Here's how the part is built. I have some questions about the finished solid (model axes, mm). Face numbers are marked on the shaded views. A direction names the side the tool comes from. Round coordinates to 2 decimals unless told otherwise and drop trailing zeros. Order: outer loops, then holes, each group sorted by start corner. A loop starts at its lowest first (then second) coordinate and runs counter-clockwise, first axis right, second up.
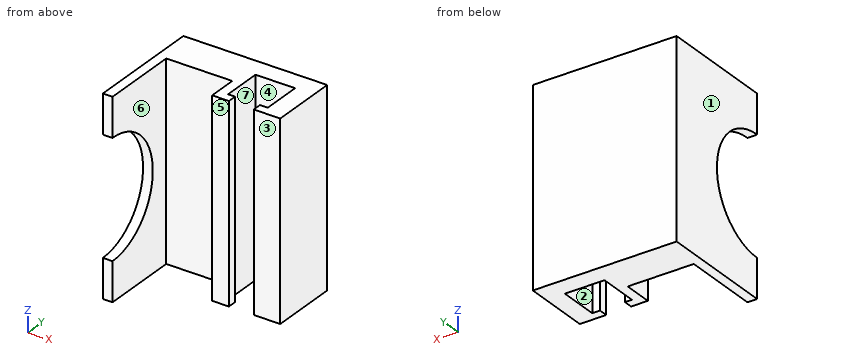
Autodesk Inventor part; units mm, degrees
ref_plane "YZ Plane" through (0, 0, 0) normal (1, 0, 0) x (0, 1, 0)
ref_plane "XZ Plane" through (0, 0, 0) normal (0, 1, 0) x (-1, 0, 0)
ref_plane "XY Plane" through (0, 0, 0) normal (0, 0, 1) x (1, 0, 0)
sketch "Skizze1" plane through (0, 0, 0) normal (0, 0, 1) x (1, 0, 0)
  line L0 (0, 0) -> (22, 0)
  line L1 (22, 0) -> (22, 10)
  line L2 (22, 10) -> (0, 10)
  line L3 (0, 10) -> (0, 0)
  dimension "d0" = 22
  dimension "d1" = 10
extrude "Extrusion1" add sketch "Skizze1" along normal blind 50
sketch "Skizze3" plane through (22, 0, 0) normal (1, 0, 0) x (0, 0, -1)
  line L0 (-50, 0) -> (-50, 10)
  line L1 (0, 0) -> (0, 10)
  line L2 (-50, 10) -> (0, 10)
  line L3 (0, 10) -> (0, 5)
  line L4 (0, 5) -> (-50, 5)
  line L5 (-50, 5) -> (-50, 10)
extrude "Extrusion2" add sketch "Skizze3" along normal blind 15
sketch "Skizze4" plane through (22, 5, 0) normal (0, -1, 0) x (1, 0, 0)
  line L0 (-22, 50) -> (15, 50)
  line L1 (15, 50) -> (10.2, 50)
  line L2 (10.2, 50) -> (10.2, 0)
  line L3 (10.2, 0) -> (15, 0)
  line L4 (15, 0) -> (15, 50)
  line L5 (0, 0) -> (0, 50)
  point P0 (-22, 0)
  dimension "d6" = 10.2
extrude "Extrusion3" add sketch "Skizze4" along normal blind 5
sketch "Skizze5" plane through (0, 0, 0) normal (0, -1, 0) x (1, 0, 0)
  line L0 (22, 0) -> (22, 50)
  line L1 (22, 50) -> (17, 50)
  line L2 (17, 50) -> (17, 0)
  line L3 (17, 0) -> (22, 0)
  line L4 (22, 0) -> (22, 50)
  line L5 (32.2, 50) -> (32.2, 0)
  line L6 (37, 0) -> (37, 50)
  line L7 (32.2, 50) -> (37, 50)
  line L8 (37, 50) -> (37, 0)
  line L9 (37, 0) -> (32.2, 0)
  line L10 (32.2, 0) -> (32.2, 50)
  point P0 (0, 0)
  dimension "d9" = 5
extrude "Extrusion4" add sketch "Skizze5" along normal blind 10
sketch "Skizze6" plane through (32.2, 5, 0) normal (-1, 0, 0) x (0, 0, 1)
  line L0 (50, 5) -> (50, -15)
  line L1 (0, 5) -> (0, -15)
  line L2 (50, -15) -> (0, -15)
  line L3 (0, -15) -> (0, -10.2)
  line L4 (0, -10.2) -> (50, -10.2)
  line L5 (50, -10.2) -> (50, -15)
  point P0 (0, -5)
  point P1 (0, -15)
  point P2 (50, -10.2)
  dimension "d12" = 4.8
extrude "Extrusion5" add sketch "Skizze6" along normal blind 2
ref_plane "Arbeitsebene1" through (27, 0, 0) normal (-1, 0, 0) x (0, 0, 1)
mirror "Spiegeln1" about plane through (27, 0, 0) normal (-1, 0, 0) of "Extrusion5"
sketch "Skizze7" plane through (0, -10, 0) normal (0, -1, 0) x (1, 0, 0)
  line L0 (0, 50) -> (37, 50)
  line L1 (17, 0) -> (17, 50)
  line L2 (37, 50) -> (17, 50)
  line L3 (17, 50) -> (17, 0)
  line L4 (17, 0) -> (37, 0)
  line L5 (37, 0) -> (37, 50)
  point P0 (0, 0)
extrude "Extrusion6" cut sketch "Skizze7" against normal blind 2.5
sketch "Skizze8" plane through (0, 0, 0) normal (-1, 0, 0) x (0, 0, 1)
  point P0 (0, 0)
sketch "Skizze9" plane through (0, 0, 0) normal (-1, 0, 0) x (0, 0, 1)
  line L0 (50, -20) -> (0, -20)
  line L1 (0, -20) -> (0, 30)
  line L2 (0, 30) -> (50, 30)
  line L3 (50, 30) -> (50, -20)
  line L4 (0, 0) -> (50, 0)
  line L5 (50, 10) -> (50, 0)
  point P0 (50, 5)
  dimension "d17" = 50
  dimension "d18" = 50
  dimension "d19" = 20
  dimension "d20" = 0
extrude "Extrusion7" add sketch "Skizze9" against normal blind 2.5
sketch "Skizze10" plane through (0, -20, 0) normal (-1, 0, 0) x (0, 0, 1)
  circle A0 centre (25, 0) radius 15
  line L0 (0, 0) -> (50, 0)
  point P0 (0, 20)
  point P1 (25, 0)
  point P2 (10, 0)
  point P3 (40, 0)
  dimension "d23" = 30
extrude "Extrusion8" cut sketch "Skizze10" against normal blind 2.5 contours L0 A0 picked at (21.7322, 7.6351)
sketch "Skizze11" plane through (17, 0, 0) normal (-1, 0, 0) x (0, 0, 1)
  line L0 (0, -7.5) -> (50, -7.5)
  line L1 (0, 0) -> (0, -7.5)
  line L2 (50, -7.5) -> (0, -7.5)
  line L3 (0, -7.5) -> (0, 0)
  line L4 (0, 0) -> (50, 0)
  line L5 (50, 0) -> (50, -7.5)
extrude "Extrusion9" cut sketch "Skizze11" against normal blind 2.5
sketch "Skizze12" plane through (2.5, 0, 0) normal (1, 0, 0) x (0, 0, -1)
  line L0 (-50, 10) -> (-50, -7.5)
  line L1 (0, 30) -> (0, -20)
  line L2 (-50, 10) -> (0, 10)
  line L3 (0, 10) -> (0, 30)
  line L4 (0, 30) -> (-50, 30)
  line L5 (-50, 30) -> (-50, 10)
  point P0 (0, 0)
  point P1 (0, 10)
extrude "Extrusion10" cut sketch "Skizze12" against normal blind 10
properties part number "Schiene"
1. If we section it at C-C, the plane z = 34: Write out the boundary of the cut face in (x, y), and give its area (3 significant figures).
Evaluation:
outline: (0, -8) - (2.5, -8) - (2.5, 0) - (19.5, 0) - (19.5, -7.5) - (23.8, -7.5) - (23.8, -5.2) - (22, -5.2) - (22, 5) - (32.2, 5) - (32.2, -5.2) - (30.2, -5.2) - (30.2, -7.5) - (37, -7.5) - (37, 10) - (0, 10) - close
area: 402 mm2
2. I'm going to push flat-ended pins straight in: P1, Ø5, axis at x = 29, z = 23, coming from the -Y side; P2, Ø5, axis at x = 9.5, z = 20, coming from the -Y side. Where does each tip first touch, or does it pass through?
Evaluation:
P1: stops at y = -7.5
P2: stops at y = 0
3. I need wall thicknesses on probe 1 along X at (y, z) = (-7, 4); probe 2 along X at (y, z) = (3, 14); probe 3 along Y at (x, z) = (22.5, 14). Which ranges of each line are inside material? Lowest first, please.
Evaluation:
probe 1: x = 0 to 2.5, 19.5 to 23.8, 30.2 to 37
probe 2: x = 0 to 22, 32.2 to 37
probe 3: y = -7.5 to -5.2, 5 to 10
4. If we mould it in two halves opening along Y, with no side actions, what happens to the marked faces 1, 2, 3 and 4? For each: released by +Y, released by -Y, zero draft, split by the parting line, or undercut.
Evaluation:
face 1: zero draft
face 2: undercut
face 3: released by -Y
face 4: undercut
5. On a 3-axis mill with a long thin cutter (end or side, diameter ignored), from which of +Z, -Z, +X, -X, +Y, -Y can I reach the whole of each face in a straight line? I mean the marked faces 5, 6 and 7. Say none if no direction works.
Evaluation:
face 5: +Z, -Z, +X, -Y
face 6: +Z, -Z, -Y
face 7: +Z, -Z
6. If we section it at B-B, the plane y = 4: Write out the boundary of the cut face in (x, z), and give its area (3 significant figures).
Evaluation:
outline: (0, 0) - (22, 0) - (22, 50) - (0, 50) - close; (32.2, 0) - (37, 0) - (37, 50) - (32.2, 50) - close
area: 1,340 mm2
7. If we section it at D-D, the plane z = 25: Write out the boundary of the cut face in (x, y).
Evaluation:
outline: (0, -5) - (2.5, -5) - (2.5, 0) - (19.5, 0) - (19.5, -7.5) - (23.8, -7.5) - (23.8, -5.2) - (22, -5.2) - (22, 5) - (32.2, 5) - (32.2, -5.2) - (30.2, -5.2) - (30.2, -7.5) - (37, -7.5) - (37, 10) - (0, 10) - close
8. If we section it at A-A, the plane y = -3.75: Write out the boundary of the cut face in (x, z), and give its area (3 significant figures).
Evaluation:
outline: (0, 0) - (2.5, 0) - (2.5, 50) - (0, 50) - close; (19.5, 0) - (22, 0) - (22, 50) - (19.5, 50) - close; (32.2, 0) - (37, 0) - (37, 50) - (32.2, 50) - close
area: 490 mm2
